from build123d import *

# Parameters (mm, degrees)
F0_W      = 184.7751736641
F0_H      = 103.2142341137
F1_DEPTH  = 74.6144801378
F3_DEPTH  = 18.3417294174
F5_DEPTH  = 18.8233163208
F7_DEPTH  = 140.3802798519
F8_R      = 12.5990656268
F9_DEPTH  = 74.6154801378
F10_R     = 13.6743893785
F11_DEPTH = 74.6154801378


with BuildPart() as f1:
    # F0 (on Top) → F1 (new body)
    with BuildSketch(Plane.XY):
        with Locations((0, -36.26935184)):
            Rectangle(F0_W, F0_H)
    extrude(amount=F1_DEPTH)

    # F2 (on face) → F3 (join)
    with BuildSketch(Plane.XZ.offset(87.8764688969)):
        with BuildLine():
            Line((44.8529869318, 74.6144801378), (-39.6928861737, 74.6144801378))
            ThreePointArc((-39.6928861737, 74.6144801378), (2.580050379, 40.7354876043), (44.8529869318, 74.6144801378))
        make_face()
    extrude(amount=F3_DEPTH)

    # F4 (on face) → F5 (join)
    with BuildSketch(Plane(origin=(0, 15.3377652168, 0), x_dir=(-1, 0, 0), z_dir=(0, 1, 0))):
        with BuildLine():
            Line((39.1467735171, 74.6144801378), (-43.5126498342, 74.6144801378))
            ThreePointArc((-43.5126498342, 74.6144801378), (-2.1829381585, 41.0193828263), (39.1467735171, 74.6144801378))
        make_face()
    extrude(amount=F5_DEPTH)

    # F6 (on face) → F7 (cut, through all)
    with BuildSketch(Plane.XZ.offset(106.2181983143)):
        with BuildLine():
            Line((29.8108495772, 74.6144801378), (-23.8135512918, 74.6144801378))
            ThreePointArc((-23.8135512918, 74.6144801378), (2.9986491427, 53.4687918706), (29.8108495772, 74.6144801378))
        make_face()
    extrude(amount=-F7_DEPTH, mode=Mode.SUBTRACT)

    # F8 (on face) → F9 (cut, through all)
    with BuildSketch(Plane.XY.offset(74.6144801378)):
        with Locations((-75.3057301044, -31.1868041754)):
            Circle(F8_R)
    extrude(amount=-F9_DEPTH, mode=Mode.SUBTRACT)

    # F10 (on face) → F11 (cut, through all)
    with BuildSketch(Plane.XY.offset(74.6144801378)):
        with Locations((74.2485821247, -31.1318598688)):
            Circle(F10_R)
    extrude(amount=-F11_DEPTH, mode=Mode.SUBTRACT)


solid = f1.part
Can you work these out from the model? Positions are in its coordinate system, mm. A direction names the side the tool comes from. Give positions to 0.01 mm unless a question says otherwise; leave off trailing zeros. Write each loop counter-clockwise with the first axis right and the second up, starting at its lowest first coordinate (ties: lowest second). Pieces come first, ordered by that corner, then holes. Notation, with made-up numbers: M -32.5,0.5 L 20.5,0.5 A11 cw 20.5,19.5 Z; hole C 74,51.5 d5. An arc over 180 degrees is marked long. Answer in a Markdown table with one row per item. Add a question column.
Item 1: On a 3-axis mill with a long thin cutter (end or side, diameter ignored), from which of +Z, -Z, +X, -X, +Y, -Y can I reach the whole of each face in a straight line? I mean faces 1 (the flat face through (-1, -87.876, 37)), 2 (the flat face through (60.7, -35, 74.614)), 3 (the cylindrical face through (2.99, 24.618, 41.027)). Say none if no direction works.
Item 2: Imagine slicing it at D-D, the plane y = -78. Write out the boundary of the cut face in (x, z).
Item 3: Imagine slicing it at B-B, the plane x = -66.5. Write out the boundary of the cut face in (y, z).
Item 4: Please list where these lines run through material, in increasing order: L1, parallel to X at y = -31, z = 35; L2, parallel to X at y = -38, z = 70.5; L3, parallel to Y at x = 46, z = 16.5.
Item 5: For pin 1 Ø1.5 at (x, y) = (31, -88.5) entering from -Z; pin 2 Ø8 at (x, z) = (72, 7.5) entering from +Y, each with a flat end and sliding along its axis, tell me the tip position at first contact or that it passes through.
Item 6: Imagine slicing it at A-A, the plane z = 64. Write out the boundary of the cut face in (x, y), plus the area to 3 significant figures.
Item 7: Imagine slicing it at C-C, the plane y = -23. Write out the boundary of the cut face in (x, z), plus the area to 3 significant figures.
Item 8: We'd pull the mould along X, two halves only. Please class faces 4 (the cylindrical face through (1.761, -96.919, 40.743)), 5 (the cylindrical face through (2.483, -37.011, 53.474)), 6 (the flat face through (2, -106.218, 50)): released by +X, released by -X, zero draft, split by the parting line, or undercut.
Evaluation:
| question | item | result |
|---|---|---|
| 1 | face 1 | -Z, -Y |
| 1 | face 2 | +Z, +X, -X, +Y, -Y |
| 1 | face 3 | -Z, +Y |
| 2 | outline | M -92.39,0 L 92.39,0 L 92.39,74.61 L 29.81,74.61 A27.57 cw -23.81,74.61 L -92.39,74.61 Z |
| 3 | outline | M -87.88,0 L -40.2,0 L -40.2,74.61 L -87.88,74.61 Z; M -22.18,0 L 15.34,0 L 15.34,74.61 L -22.18,74.61 Z |
| 4 | L1 | x = -92.39 to -87.9, -62.71 to 60.57, 87.92 to 92.39 |
| 4 | L2 | x = -92.39 to -85.9, -64.71 to -22.48, 28.48 to 62.42, 86.07 to 92.39 |
| 4 | L3 | y = -87.88 to 15.34 |
| 5 | pin 1 | stops at z = 0 |
| 5 | pin 2 | stops at y = 15.34 |
| 6 | outline | M -92.39,-87.88 L -35.81,-87.88 L -35.81,-106.22 L -18.68,-106.22 L -18.68,34.16 L -35.4,34.16 L -35.4,15.34 L -92.39,15.34 Z; M 24.67,-106.22 L 40.97,-106.22 L 40.97,-87.88 L 92.39,-87.88 L 92.39,15.34 L 39.76,15.34 L 39.76,34.16 L 24.67,34.16 Z; hole C -75.31,-31.19 d25.2; hole C 74.25,-31.13 d27.35 |
| 6 | area | 14,700 mm² |
| 7 | outline | M -92.39,0 L -84.88,0 L -84.88,74.61 L -92.39,74.61 Z; M -65.73,0 L 63.25,0 L 63.25,74.61 L 29.81,74.61 A27.57 cw -23.81,74.61 L -65.73,74.61 Z; M 85.24,0 L 92.39,0 L 92.39,74.61 L 85.24,74.61 Z |
| 7 | area | 9,870 mm² |
| 8 | face 4 | split by the parting line |
| 8 | face 5 | undercut |
| 8 | face 6 | zero draft |
